Autodesk Inventor part; units mm, degrees
ref_plane "YZ Plane" through (0, 0, 0) normal (1, 0, 0) x (0, 1, 0)
ref_plane "XZ Plane" through (0, 0, 0) normal (0, 1, 0) x (-1, 0, 0)
ref_plane "XY Plane" through (0, 0, 0) normal (0, 0, 1) x (1, 0, 0)
sketch "Boceto1" plane through (0, 0, 0) normal (0, 1, 0) x (-1, 0, 0)
  line L0 (6.1283, -21.2541) -> (6.1283, -85.7541)
  line L1 (6.1283, -85.7541) -> (-253.3717, -85.7541)
  line L2 (6.1283, -21.2541) -> (-253.3717, -21.2541)
  line L3 (-253.3717, -21.2541) -> (-253.3717, -85.7541)
  circle A0 centre (-127.3717, -61.2541) radius 4
  circle A1 centre (-10.3717, -61.2541) radius 4
  circle A2 centre (-68.8717, -61.2541) radius 8
  circle A3 centre (-35.3717, -79.2541) radius 1.5
  circle A4 centre (-43.3717, -79.2541) radius 1.5
  circle A5 centre (-28.8717, -53.2541) radius 3
  circle A6 centre (-173.3717, -67.7541) radius 3
  circle A7 centre (-173.3717, -39.2541) radius 3
  dimension "d0" = 64.5
  dimension "d22" = 8
  dimension "d23" = 8
  dimension "d27" = 16
  dimension "d103" = 58.5
  dimension "d104" = 117
  dimension "d105" = 3
  dimension "d106" = 3
  dimension "d115" = 6.5
  dimension "d121" = 259.5
  dimension "d122" = 126
  dimension "d128" = 6
  dimension "d129" = 35
  dimension "d130" = 32
  dimension "d131" = 6
  dimension "d132" = 6
  dimension "d133" = 80
  dimension "d134" = 18
  dimension "d135" = 80
  dimension "d136" = 18
  dimension "d143" = 40
  dimension "d144" = 40
  dimension "d145" = 40
  dimension "d149" = 8
  dimension "d150" = 41.5
extrude "Extrusion3" add sketch "Boceto1" along normal blind 12
sketch "Sketch2" plane through (0, 12, 0) normal (0, 1, 0) x (1, 0, 0)
  circle A0 centre (6.3717, 26.2541) radius 3
  line L0 (-6.1283, 21.2541) -> (253.3717, 21.2541)
  line L1 (-6.1283, 85.7541) -> (-6.1283, 21.2541)
  circle A1 centre (31.3717, 26.2541) radius 3
  circle A2 centre (218.3717, 71.2541) radius 3
  circle A3 centre (238.3717, 71.2541) radius 3
  circle A4 centre (218.3717, 36.2541) radius 3
  circle A5 centre (238.3717, 36.2541) radius 3
  line L2 (253.3717, 21.2541) -> (253.3717, 85.7541)
  line L3 (253.3717, 85.7541) -> (-6.1283, 85.7541)
  point P0 (253.3717, 20.7541)
  point P1 (-7.6283, 85.7541)
  dimension "d84" = 6
  dimension "d85" = 5
  dimension "d86" = 12.5
  dimension "d87" = 6
  dimension "d88" = 25
  dimension "d91" = 6
  dimension "d92" = 6
  dimension "d93" = 6
  dimension "d94" = 6
  dimension "d95" = 15
  dimension "d98" = 15
  dimension "d99" = 15
  dimension "d100" = 20
  dimension "d101" = 20
  dimension "d146" = 35
  dimension "d147" = 35
  dimension "d148" = 15
extrude "Extrusion4" cut sketch "Sketch2" against normal blind 25 contours A0 | A1 | A2 | A3 | A4 | A5
thread "Thread1"
thread "Thread2"
thread "Rosca3"
thread "Rosca4"
thread "Rosca5"
properties part number "Columna Izquierda" material "Aluminum 6061"
The listing builds one solid part. Answer for the finished solid, in the listing's coordinates (mm). Coordinates: 2 decimals unless noted, no trailing zeros. Put each result on its own line as item: value.
1. Determine the mould class of faces 1 (the face through (34.23, 6.08, -27.16)), 2 (the face through (125, 12, -53)), 3 (the face through (235.375, 6.084, -36.386)), 4 (the face through (122, 6, -85.754)) for opening direction Z: pulls with the +Z half, pulls with the -Z half, needs draft (parallel to the pull), parting line crosses it, or undercut.
Answer sheet:
face 1: undercut
face 2: needs draft
face 3: undercut
face 4: pulls with the -Z half
2. The part is cut by section A-A on y = 5.5. State how many separate pieces and enclosed holes the cut face has, plus the area to 3 significant figures.
Answer sheet:
separate pieces: 1
enclosed holes: 14
area: 16,200 mm^2
3. Find the intervals of material crossed by line 1 along X through (y, z) = (10, -28); line 2 along Z through (x, y) = (43, 5); line 3 along Z through (x, y) = (240, 4.75), in increasing order. Write a range as from..to.
Answer sheet:
line 1: x = -6.13..3.93, 8.81..28.93, 33.81..253.37
line 2: z = -85.75..-80.71, -77.8..-21.25
line 3: z = -85.75..-73.77, -68.73..-38.77, -33.73..-21.25
